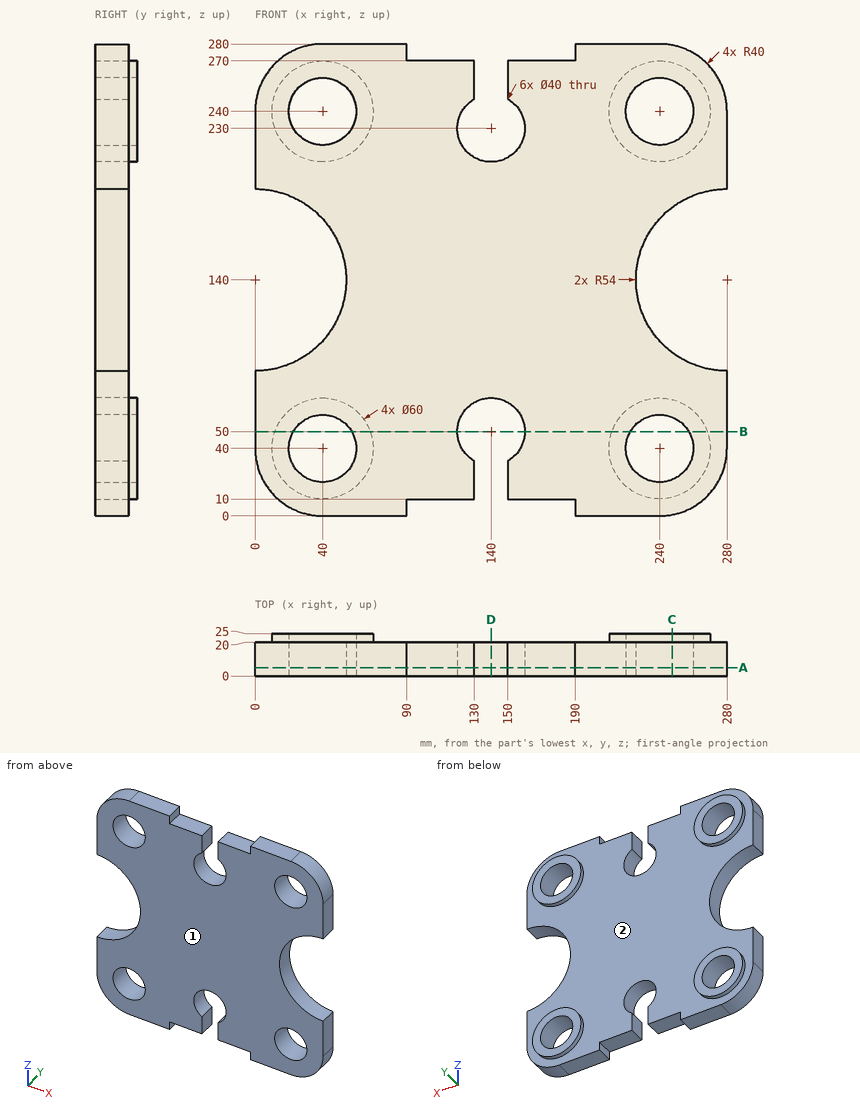
Here's the drawing with two shaded views (mm, measured from the low corner). I have some questions. Give positions to 0.01 mm unless a question says otherwise; leave off trailing zeros. Write each loop counter-clockwise with the first axis right and the second up, starting at its lowest first coordinate (ties: lowest second). Pieces come first, ordered by that corner, then holes. Notation, with made-up numbers: (10, -37.75) -> (37, -37.75) arc R21 cw to (37, -28.75) -> close; hole circle Ø5 at (-2.5, 33). An arc over 180 degrees is marked (long way). Answer as a JSON object with one key per item and string values. Group by question number.
Item 1: Suppose I cut it at C-C (x = 247.5). Please give me the cut outline in (y, z), plus the area to 3 significant figures.
Item 2: Suppose I cut it at A-A (y = 5). State how many separate pieces and enclosed holes the cut face has, plus the area to 3 significant figures.
Item 3: Suppose I cut it at B-B (z = 50). Please give me the cut outline in (x, y), plus the area to 3 significant figures.
Item 4: I'm going to push flat-ended pins straight in: P1, Ø1.5, axis at y = 8, z = 113, coming from the -X side; P2, Ø5, axis at y = 6, z = 277, coming from the +X side; P3, Ø24, axis at x = 240, z = 240, coming from the -Y side; P4, Ø6, axis at y = 11.5, z = 23, coming from the +X side. Where does each tip first touch, or does it pass through?
Item 5: Please list where these lines run through material, in increasing order: line 1 (X direction, y = 13.25, z = 240); line 2 (Z direction, x = 25, y = 12); line 3 (Z direction, x = 158, y = 12.5). Write a range as [from, to].
Item 6: We'd pull the mould along X, two halves only. Please class the marked faces 1 and 2: +X half, -X half, draft (parallel to the pull), parting line (faces both ways), or undercut.
Item 7: Suppose I cut it at D-D (x = 140). Please give me the cut outline in (y, z), plus the area to 3 significant figures.
Findings:
{
 "1": {"outline": "(0, 0.71) -> (20, 0.71) -> (20, 10.95) -> (25, 10.95) -> (25, 21.46) -> (0, 21.46) -> close; (0, 58.54) -> (25, 58.54) -> (25, 69.05) -> (20, 69.05) -> (20, 96.88) -> (0, 96.88) -> close; (0, 183.12) -> (20, 183.12) -> (20, 210.95) -> (25, 210.95) -> (25, 221.46) -> (0, 221.46) -> close; (0, 258.54) -> (25, 258.54) -> (25, 269.05) -> (20, 269.05) -> (20, 279.29) -> (0, 279.29) -> close", "area": "2,570 mm²"},
 "2": {"separate pieces": "1", "enclosed holes": "4", "area": "57,500 mm²"},
 "3": {"outline": "(0, 0) -> (22.68, 0) -> (22.68, 25) -> (11.72, 25) -> (11.72, 20) -> (0, 20) -> close; (57.32, 0) -> (120, 0) -> (120, 20) -> (68.28, 20) -> (68.28, 25) -> (57.32, 25) -> close; (160, 0) -> (222.68, 0) -> (222.68, 25) -> (211.72, 25) -> (211.72, 20) -> (160, 20) -> close; (257.32, 0) -> (280, 0) -> (280, 20) -> (268.28, 20) -> (268.28, 25) -> (257.32, 25) -> close", "area": "3,630 mm²"},
 "4": {"P1": "stops at x = 46.32", "P2": "stops at x = 260.24", "P3": "passes through", "P4": "stops at x = 277.47"},
 "5": {"line 1": "x = [0, 20], [60, 122.68], [157.32, 220], [260, 280]", "line 2": "z = [2.92, 26.77], [53.23, 92.14], [187.86, 226.77], [253.23, 277.08]", "line 3": "z = [10, 41.28], [58.72, 221.28], [238.72, 270]"},
 "6": {"face 1": "draft", "face 2": "undercut"},
 "7": {"outline": "(0, 70) -> (20, 70) -> (20, 210) -> (0, 210) -> close", "area": "2,800 mm²"}
}
